Design review of the part built by this model. Coordinates are the model's own, in mm. A direction names the side the tool comes from. Give positions to 0.01 mm unless a question says otherwise; leave off trailing zeros. Loops run counter-clockwise (first coordinate to the right, second up) from the corner with the lowest first, then second, coordinate; pieces in that order, holes last.
from build123d import *

# Parameters (mm, degrees)
BOSS_EXTRUDE1_DEPTH = 1.5
SKETCH2_R           = 1
CUT_EXTRUDE1_DEPTH  = 5
CHAMFER1_SIZE       = 2


with BuildPart() as part:
    # Sketch1 → Boss-Extrude1 (new body)
    with BuildSketch(Plane.XY):
        with BuildLine():
            Line((-4, -100), (4, -100))
            Line((4, -100), (4, -65.477225575))
            ThreePointArc((4, -65.477225575), (3.414213562, -64.063012013), (2, -63.477225575))
            Line((2, -63.477225575), (-1, -63.477225575))
            Line((-1, -63.477225575), (-1, -56.522774425))
            Line((-1, -56.522774425), (2, -56.522774425))
            ThreePointArc((2, -56.522774425), (4, -54.522774425), (2, -52.522774425))
            Line((2, -52.522774425), (-4, -52.522774425))
            Line((-4, -52.522774425), (-4, -100))
        make_face()
    extrude(amount=BOSS_EXTRUDE1_DEPTH)

    # Sketch2 → Cut-Extrude1 (cut)
    with BuildSketch(Plane.XY.offset(1.5)):
        with Locations((-1.5, -97)):
            Circle(SKETCH2_R)
        with Locations((1.5, -94)):
            Circle(SKETCH2_R)
        with Locations((-1.5, -91)):
            Circle(SKETCH2_R)
        with Locations((-1.5, -85)):
            Circle(SKETCH2_R)
        with Locations((1.5, -88)):
            Circle(SKETCH2_R)
    extrude(amount=-CUT_EXTRUDE1_DEPTH, mode=Mode.SUBTRACT)

    # Chamfer1
    chamfer1_edges = [part.edges().sort_by_distance(p)[0] for p in [
        (-4, -52.522774425, 0.75),
        (-1, -56.522774425, 0.75),
        (-1, -63.477225575, 0.75),
        (4, -100, 0.75),
        (-4, -100, 0.75),
    ]]
    chamfer(chamfer1_edges, length=CHAMFER1_SIZE)


solid = part.part
Q1. Take a section at A-A (y = -88). Give the boundary of the cut face in (x, z), plus the area to 3 significant figures.
Results:
outline: (-4, 0) - (0.5, 0) - (0.5, 1.5) - (-4, 1.5) - close; (2.5, 0) - (4, 0) - (4, 1.5) - (2.5, 1.5) - close
area: 9.00 mm2
Q2. Draft analysis for pull direction Y (two halves, no side actions). For faces 3 (the face through (1.5, -63.477, 0.7)), 4 (the face through (0, -100, 1)), 5 (the face through (0, -76, 1.5)), state which applies: pulls with the +Y half, pulls with the -Y half, needs draft (parallel to the pull), parting line crosses it, or undercut.
Results:
face 3: undercut
face 4: pulls with the -Y half
face 5: needs draft
Q3. Tool access review of faces 1 (the face through (-1, -60, 1)), 2 (the face through (-1.04, -97.89, 0.76)): name each direction out of +Z, -Z, +X, -X, +Y, -Y from which nothing blocks a thin tool from reaching the whole face with its end or side.
Results:
face 1: +Z, -Z, +X
face 2: +Z, -Z
Q4. Insertion check: pin 1 (2.5 mm diameter, centred on x = -1.5, y = -85, fed in from +Z). The pin has a flat end and moves straight along its axis. Give the tip position at first contact, or say it passes through.
Results:
pin 1: stops at z = 1.5
Q5. Take a section at C-C (z = 0.9). Give the boundary of the cut face in (x, y), plus the area to 3 significant figures.
Results:
outline: (-4, -98) - (-2, -100) - (2, -100) - (4, -98) - (4, -65.48) arc R2 ccw to (2, -63.48) - (1, -63.48) - (-1, -61.48) - (-1, -58.52) - (1, -56.52) - (2, -56.52) arc R2 ccw to (2, -52.52) - (-2, -52.52) - (-4, -54.52) - close; hole circle Ø2 at (-1.5, -97); hole circle Ø2 at (-1.5, -91); hole circle Ø2 at (-1.5, -85); hole circle Ø2 at (1.5, -94); hole circle Ø2 at (1.5, -88)
area: 325 mm2
Q6. Take a section at D-D (x = 3.5). Give the boundary of the cut face in (y, z), plus the area to 3 significant figures.
Results:
outline: (-98.5, 0) - (-64.15, 0) - (-64.15, 1.5) - (-98.5, 1.5) - close; (-55.85, 0) - (-53.2, 0) - (-53.2, 1.5) - (-55.85, 1.5) - close
area: 55.5 mm2
Q7. Take a section at B-B (x = 1.5). Give the boundary of the cut face in (y, z).
Results:
outline: (-100, 0) - (-95, 0) - (-95, 1.5) - (-100, 1.5) - close; (-93, 0) - (-89, 0) - (-89, 1.5) - (-93, 1.5) - close; (-87, 0) - (-63.48, 0) - (-63.48, 1.5) - (-87, 1.5) - close; (-56.52, 0) - (-52.52, 0) - (-52.52, 1.5) - (-56.52, 1.5) - close
Q8. Wall thickness on line 1 (Y direction, x = -1.5, z = 1.1); line 2 (Y direction, x = 1.5, z = 0.6); line 3 (X direction, y = -88, z = 1.15): over which ranges is each line inside the solid? List them lowest first.
Results:
line 1: y = -100 to -98, -96 to -92, -90 to -86, -84 to -52.52
line 2: y = -100 to -95, -93 to -89, -87 to -63.48, -56.52 to -52.52
line 3: x = -4 to 0.5, 2.5 to 4
